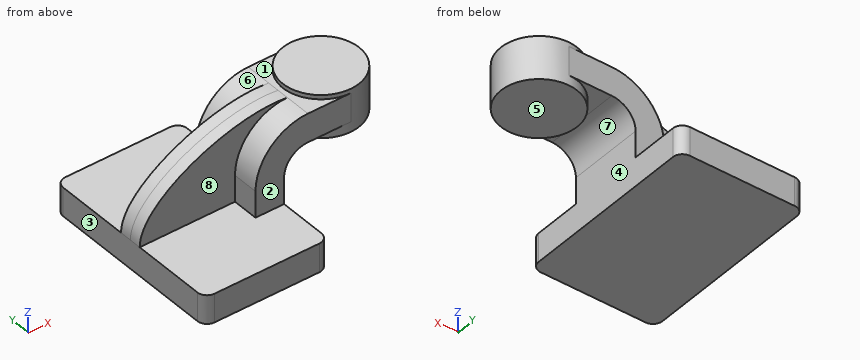
```python
from build123d import *

# Parameters (mm, degrees)
F1_DEPTH = 63.5
F2_DEPTH = 25.4
F3_DEPTH = 7.9375
F5_R     = 6.35


with BuildPart() as f1:
    # F0 (on Front) → F1 (new body, symmetric)
    with BuildSketch(Plane.XZ):
        Polygon((-41.275, -9.525), (41.275, -9.525), (41.275, 9.525), (22.225, 9.525), (-41.275, 9.525), align=None)
    extrude(amount=F1_DEPTH, both=True)

    # F0 (on Front) → F2 (join, symmetric)
    with BuildSketch(Plane.XZ):
        with BuildLine():
            Line((22.225, 9.525), (41.275, 9.525))
            Line((41.275, 9.525), (41.275, 27.0002))
            ThreePointArc((41.275, 27.0002), (45.9246798487, 38.2255201513), (57.15, 42.8752))
            Line((57.15, 42.8752), (60.325, 42.8752))
            Line((60.325, 42.8752), (60.325, 61.9252))
            Line((60.325, 61.9252), (57.15, 61.9252))
            ThreePointArc((57.15, 61.9252), (32.4542956671, 51.6959043329), (22.225, 27.0002))
            Line((22.225, 27.0002), (22.225, 9.525))
        make_face()
        Polygon((85.725, 61.9252), (60.325, 61.9252), (60.325, 42.8752), (85.725, 42.8752), (85.725, 50.4787749963), align=None)
    extrude(amount=F2_DEPTH, both=True)

    # F0 (on Front) → F3 (join, symmetric)
    with BuildSketch(Plane.XZ):
        with BuildLine():
            add(Edge.make_bspline(
                [(-41.275, 9.525), (-41.2498526275, 38.3011959493), (19.6118596941, 66.9183731079), (57.15, 61.9252)],
                knots=[0, 0, 0, 0, 111.5045361635, 111.5045361635, 111.5045361635, 111.5045361635], degree=3))
            Line((-41.275, 9.525), (22.225, 9.525))
            Line((22.225, 9.525), (22.225, 27.0002))
            ThreePointArc((22.225, 27.0002), (32.4542956671, 51.6959043329), (57.15, 61.9252))
        make_face()
    extrude(amount=F3_DEPTH, both=True)

    # F0 (on Front) → F4 (revolve)
    with BuildSketch(Plane.XZ):
        Polygon((85.725, 64.7662749963), (85.725, 61.9252), (85.725, 50.4787749963), (85.725, 42.8752), (85.725, 36.1912749963), (111.125, 36.1912749963), (111.125, 64.7662749963), align=None)
    revolve(axis=Axis((85.725, 0, 50.4787749963), (0, 0, -1)))

    # F5
    f5_edges = [f1.edges().sort_by_distance(p)[0] for p in [
        (-41.275, -63.5, 0),
        (41.275, -63.5, 0),
        (41.275, 63.5, 0),
        (-41.275, 63.5, 0),
    ]]
    fillet(f5_edges, radius=F5_R)


solid = f1.part
```
Check sheet for the modelled part. Datum: model origin and axes. Units: mm. Face numbers are marked on the shaded views. A direction names the side the tool comes from. Round coordinates to 2 decimals unless told otherwise and drop trailing zeros. Order: outer loops, then holes, each group sorted by start corner. A loop starts at its lowest first (then second) coordinate and runs counter-clockwise, first axis right, second up. Notation, with made-up numbers: (-30, -20) - (-20, -20) arc R13 cw to (-20, -13) - close; hole circle Ø4 at (-12.5, -19.75). An arc over 180 degrees is marked (long way). Write item = value, one per line.
Q1. Section check B-B (y = -18). Record the boundary of the cut face in (x, z) (3 decimals), and give its area (3 significant figures).
Computed:
outline = (-41.275, -9.525) - (41.275, -9.525) - (41.275, 27) arc R15.875 cw to (57.15, 42.875) - (67.804, 42.875) - (67.804, 36.191) - (103.646, 36.191) - (103.646, 64.766) - (67.804, 64.766) - (67.804, 61.925) - (57.15, 61.925) arc R34.925 ccw to (22.225, 27) - (22.225, 9.525) - (-41.275, 9.525) - close
area = 3,890 mm^2
Q2. Thickness scan on line 1 along Y through (x, z) = (-27, 34.5); line 2 along Z through (x, y) = (7, -21) (3 decimals); line 3 along X through (y, z) = (-53.5, 8.5) (3 decimals). Record the ranges inside material, lowest first.
Computed:
line_1 = -7.94 to 7.94
line_2 = -9.525 to 9.525
line_3 = -41.275 to 41.275
Q3. Draft check along X on the marked faces 1, 2, 3 and 4. Enter one of: pulls with the +X half, pulls with the -X half, needs draft (parallel to the pull), parting line crosses it, or undercut.
Computed:
face_1 = undercut
face_2 = needs draft
face_3 = pulls with the -X half
face_4 = pulls with the +X half
Q4. Tool access check on the marked faces 5, 6, 7 and 8. Record the directions out of +Z, -Z, +X, -X, +Y, -Y that give a thin tool (end or side, any length) a straight path to the whole face; none if there is none.
Computed:
face_5 = -Z, +X, +Y, -Y
face_6 = +Z, -X, +Y
face_7 = -Z, +Y, -Y
face_8 = +Z, -X, -Y
Q5. Section check D-D (y = 13.5). Record the boundary of the cut face in (x, z) (3 decimals).
Computed:
outline = (-41.275, -9.525) - (41.275, -9.525) - (41.275, 27) arc R15.875 cw to (57.15, 42.875) - (64.21, 42.875) - (64.21, 36.191) - (107.24, 36.191) - (107.24, 64.766) - (64.21, 64.766) - (64.21, 61.925) - (57.15, 61.925) arc R34.925 ccw to (22.225, 27) - (22.225, 9.525) - (-41.275, 9.525) - close
Q6. Section check C-C (x = 83). Record the boundary of the cut face in (y, z), and give its area (3 significant figures).
Computed:
outline = (-25.4, 42.88) - (-25.25, 42.88) - (-25.25, 36.19) - (25.25, 36.19) - (25.25, 42.88) - (25.4, 42.88) - (25.4, 61.93) - (25.25, 61.93) - (25.25, 64.77) - (-25.25, 64.77) - (-25.25, 61.93) - (-25.4, 61.93) - close
area = 1,450 mm^2
Q7. Section check A-A (z = 0). Record the boundary of the cut face in (x, y) (3 decimals), and give its area (3 significant figures).
Computed:
outline = (-41.275, -57.15) arc R6.35 ccw to (-34.925, -63.5) - (34.925, -63.5) arc R6.35 ccw to (41.275, -57.15) - (41.275, 57.15) arc R6.35 ccw to (34.925, 63.5) - (-34.925, 63.5) arc R6.35 ccw to (-41.275, 57.15) - close
area = 10,400 mm^2
Q8. Go/stop test with flat-tipped pins: pin 1 (16.5 mm diameter, centred on x = -18.5, y = 27.5, fed in from +Z) (3 decimals); pin 2 (4 mm diameter, centred on x = -20.5, y = -9.5, fed in from +Z); pin 3 (12 mm diameter, centred on x = 23.5, z = 42.5, fed in from -Y). Record where each tip stops, or that it passes through.
Computed:
pin_1 = 9.525
pin_2 = 40.61
pin_3 = -25.4
